Input: dimensioned drawing with shaded views. Units: mm. Origin: part minimum x, y, z. A direction names the side the tool comes from. Round coordinates to 2 decimals unless told otherwise and drop trailing zeros. Write each loop counter-clockwise with the first axis right and the second up, starting at its lowest first coordinate (ties: lowest second). Pieces come first, ordered by that corner, then holes. Notation, with made-up numbers: (-22.75, 50.25) - (9.25, 50.25) arc R9 ccw to (9.25, 57.25) - close; hole circle Ø7 at (23.25, 9). An arc over 180 degrees is marked (long way). Use one line per item in the form item = value.
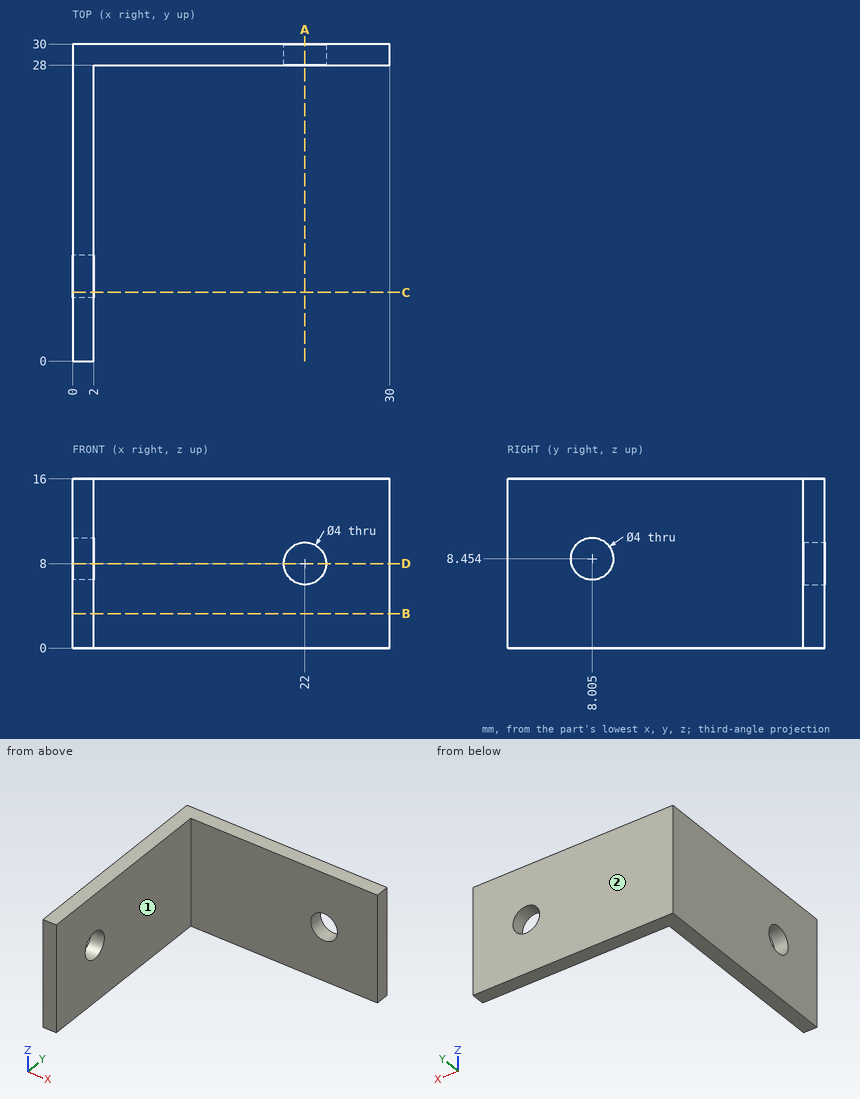
(1) Cut plane C-C on y = 6.5. Output: boundary loops of the cut face in (x, z).
Derived:
outline = (0, 0) - (2, 0) - (2, 7.14) - (0, 7.14) - close; (0, 9.77) - (2, 9.77) - (2, 16) - (0, 16) - close
(2) Cut plane B-B on z = 3.25. Output: boundary loops of the cut face in (x, y), then the cut area to 3 significant figures.
Derived:
outline = (0, 0) - (2, 0) - (2, 28) - (30, 28) - (30, 30) - (0, 30) - close
area = 116 mm^2
(3) Material intervals for L1, parallel to Z at x = 22, y = 29.15; L2, parallel to X at y = 29.25, z = 8; L3, parallel to Y at x = 8.5, z = 9.25, sorted ascending.
Derived:
L1 = 0 to 6, 10 to 16
L2 = 0 to 20, 24 to 30
L3 = 28 to 30
(4) First-contact query: pin 1 Ø1 at (x, z) = (24.5, 6) entering from -Y; pin 2 Ø12 at (x, y) = (12.5, 15.5) entering from +Z; pin 3 Ø2 at (y, z) = (20, 11) entering from +X. Flat tips, straight axial feed; report the tip coordinate or a pass-through.
Derived:
pin_1 = 28
pin_2 = through
pin_3 = 2
(5) Cut plane A-A on x = 22. Output: boundary loops of the cut face in (y, z), then the cut area to 3 significant figures.
Derived:
outline = (28, 0) - (30, 0) - (30, 6) - (28, 6) - close; (28, 10) - (30, 10) - (30, 16) - (28, 16) - close
area = 24.0 mm^2
(6) Access query for the marked faces 1 and 2. Directions: +Z, -Z, +X, -X, +Y, -Y. A direction counts if a zero-diameter tool reaches every point of the face in a straight line with its end or side. Return the directions, or none.
Derived:
face_1 = +Z, -Z, +X, -Y
face_2 = +Z, -Z, +X, -X, +Y
(7) Cut plane D-D on z = 8. Output: boundary loops of the cut face in (x, y).
Derived:
outline = (0, 0) - (2, 0) - (2, 6.06) - (0, 6.06) - close; (0, 9.95) - (2, 9.95) - (2, 28) - (20, 28) - (20, 30) - (0, 30) - close; (24, 28) - (30, 28) - (30, 30) - (24, 30) - close
